Input: part model. Units: mm. Frame: model coordinates. A direction names the side the tool comes from. Give positions to 0.01 mm unless a question says otherwise; leave off trailing zeros. Loops run counter-clockwise (first coordinate to the right, second up) from the corner with the lowest first, then second, coordinate; pieces in that order, holes last. Notation, with made-up numbers: M -7,67.5 L -3,67.5 A4 cw -3,71.5 Z; hole C 0,-22.75 d8. An arc over 180 degrees is marked long. Answer as a JSON object with one key per item and string values. Group by question number.
1) Section query B-B on z = -1.5. Return loops of the section in (x, y), plus the area to 3 significant figures.
2) Section query C-C on x = 3.58. Return loops of the section in (y, z).
3) Section query A-A on y = 10. Return loops of the section in (x, z) (3 decimals).
4) Section query D-D on y = 23. Return loops of the section in (x, z), plus the area to 3 significant figures.
5) Draft query along X for faces 5 (the flat face through (-8.8, 32.2, 5)), 6 (the cylindrical face through (-14, 34, 8)), 7 (the flat face through (-21, 23, 0)), 8 (the flat face through (-10, 23, -10)). Return one class per face: +X half, -X half, draft (parallel to the pull), parting line (faces both ways), or undercut.
6) Ray query, L1, parallel to Y at x = -11, z = 8; L2, parallel to Z at x = 3, y = 44; L3, parallel to Y at x = -11.5, z = 1.5. Return the intervals inside material, ascending.
7) First-contact query: P1, Ø1.4, axis at x = 3.5, z = 2.5, coming from the +Y side; P2, Ø16, axis at x = -11, y = 10, coming from the -Z side; P3, Ø2.5, axis at x = 3.5, z = -18, coming from the +Y side. Flat tips, straight axial feed; report the tip coordinate or a pass-through.
8) Access query for faces 1 (the flat face through (4, 0, -4)), 2 (the flat face through (-0.9, 23, -17)), 3 (the flat face through (-8.8, 12.2, 5)), 4 (the flat face through (4, 39.7, -18)). Directions: +Z, -Z, +X, -X, +Y, -Y. A direction counts if a zero-diameter tool reaches every point of the face in a straight line with its end or side. Return the directions, or none.
from build123d import *

# Parameters (mm, degrees)
SKETCH1_W                     = 42
SKETCH1_H                     = 20
BOSS_EXTRUDE1_DEPTH           = 40
SKETCH2_W                     = 21.9
SKETCH2_H                     = 15
BOSS_EXTRUDE2_DEPTH           = 40
CBORE_FOR_M5_SHCS1_AT_2_COUNT = 2
CBORE_FOR_M5_SHCS1_AT_2_PITCH = 20
BOSS_EXTRUDE3_DEPTH           = 6.5
FILLET1_R                     = 1
SKETCH8_R                     = 2.4
CUT_EXTRUDE1_DEPTH            = 3.8
SKETCH9_R                     = 1.65
CUT_EXTRUDE2_DEPTH            = 3


with BuildPart() as part:
    # Sketch1 → Boss-Extrude1 (new body)
    with BuildSketch(Plane(origin=(0, 0, 0), x_dir=(1, 0, 0), z_dir=(0, 1, 0))):
        Rectangle(SKETCH1_W, SKETCH1_H)
    extrude(amount=BOSS_EXTRUDE1_DEPTH)

    # Sketch2 → Boss-Extrude2 (add)
    with BuildSketch(Plane(origin=(0, 40, 0), x_dir=(1, 0, 0), z_dir=(0, 1, 0))):
        with Locations((10.05, 17.5)):
            Rectangle(SKETCH2_W, SKETCH2_H)
    extrude(amount=-BOSS_EXTRUDE2_DEPTH)

    # Sketch5 → CBORE for M5 SHCS1 (revolve, cut)
    with BuildSketch(Plane(origin=(-11, 30, 10), x_dir=(0, -1, 0), z_dir=(1, 0, 0))):
        Polygon((0, 0), (0, 35), (2.75, 35), (2.75, 5), (5, 5), (5, 0.020977491), (5.025, 0), align=None)
    cbore_for_m5_shcs1 = revolve(axis=Axis((-11, 30, 16.35), (0, 0, -1)), mode=Mode.SUBTRACT)

    # CBORE for M5 SHCS1 at 2: CBORE for M5 SHCS1 ×2
    with Locations(*[(0, -i * CBORE_FOR_M5_SHCS1_AT_2_PITCH, 0) for i in range(1, CBORE_FOR_M5_SHCS1_AT_2_COUNT)]):
        add(cbore_for_m5_shcs1, mode=Mode.SUBTRACT)

    # Sketch6 → Boss-Extrude3 (add)
    with BuildSketch(Plane(origin=(0, 40, 0), x_dir=(1, 0, 0), z_dir=(0, 1, 0))):
        Polygon((-21, 10), (-21, -10), (21, -10), (21, 25), (-0.9, 25), (-0.9, 10), align=None)
    extrude(amount=BOSS_EXTRUDE3_DEPTH)

    # Fillet1
    fillet1_edges = [part.edges().sort_by_distance(p)[0] for p in [
        (-0.9, 23.25, -25),
        (21, 23.25, -25),
        (-21, 23.25, -10),
        (21, 23.25, 10),
        (-21, 23.25, 10),
    ]]
    fillet(fillet1_edges, radius=FILLET1_R)

    # Sketch8 → Cut-Extrude1 (cut)
    with BuildSketch(Plane(origin=(0, 46.5, 0), x_dir=(1, 0, 0), z_dir=(0, 1, 0))):
        with Locations((3.58, 17.5)):
            Circle(SKETCH8_R)
        with Locations((3.58, -2.5)):
            Circle(SKETCH8_R)
    extrude(amount=-CUT_EXTRUDE1_DEPTH, mode=Mode.SUBTRACT)

    # Sketch9 → Cut-Extrude2 (cut)
    with BuildSketch(Plane(origin=(0, 42.7, 0), x_dir=(1, 0, 0), z_dir=(0, 1, 0))):
        with Locations((3.58, 17.5)):
            Circle(SKETCH9_R)
        with Locations((3.58, -2.5)):
            Circle(SKETCH9_R)
    extrude(amount=-CUT_EXTRUDE2_DEPTH, mode=Mode.SUBTRACT)


solid = part.part
Output:
{
 "1": {"outline": "M -21,0 L 21,0 L 21,46.5 L -21,46.5 Z; hole C -11,10 d5.5; hole C -11,30 d5.5", "area": "1,910 mm^2"},
 "2": {"outline": "M 0,-25 L 46.5,-25 L 46.5,-19.9 L 42.7,-19.9 L 42.7,-19.15 L 39.7,-19.15 L 39.7,-15.85 L 42.7,-15.85 L 42.7,-15.1 L 46.5,-15.1 L 46.5,0.1 L 42.7,0.1 L 42.7,0.85 L 39.7,0.85 L 39.7,4.15 L 42.7,4.15 L 42.7,4.9 L 46.5,4.9 L 46.5,10 L 0,10 Z"},
 "3": {"outline": "M -21,-9 A1 ccw -20,-10 L -13.75,-10 L -13.75,5 L -16,5 L -16,9.979 L -16.025,10 L -20,10 A1 ccw -21,9 Z; M -8.25,-10 L -0.9,-10 L -0.9,-24 A1 ccw 0.1,-25 L 20,-25 A1 ccw 21,-24 L 21,9 A1 ccw 20,10 L -5.975,10 L -6,9.979 L -6,5 L -8.25,5 Z"},
 "4": {"outline": "M -21,-9 A1 ccw -20,-10 L -0.9,-10 L -0.9,-24 A1 ccw 0.1,-25 L 20,-25 A1 ccw 21,-24 L 21,9 A1 ccw 20,10 L -20,10 A1 ccw -21,9 Z", "area": "1,170 mm^2"},
 "5": {"face 5": "undercut", "face 6": "undercut", "face 7": "-X half", "face 8": "draft"},
 "6": {"L1": "y = 0 to 5, 15 to 25, 35 to 46.5", "L2": "z = -25 to -19.83, -15.17 to 0.17, 4.83 to 10", "L3": "y = 0 to 7.3, 12.7 to 27.3, 32.7 to 46.5"},
 "7": {"P1": "stops at y = 39.7", "P2": "stops at z = -10", "P3": "stops at y = 42.7"},
 "8": {"face 1": "+Z, -Z, +X, -X, -Y", "face 2": "-Z, -X, +Y, -Y", "face 3": "+Z", "face 4": "+Y"}
}
